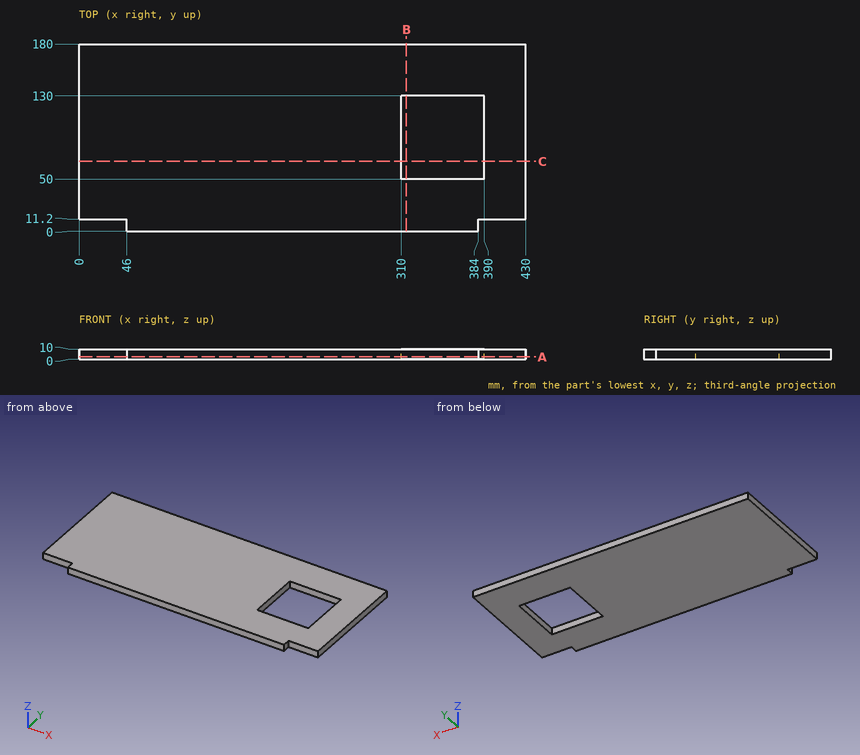
Drawing for the job (mm, zero at the part's lowest x, y, z). Give positions to 0.01 mm unless a question says otherwise; leave off trailing zeros. Order: outer loops, then holes, each group sorted by start corner. A loop starts at its lowest first (then second) coordinate and runs counter-clockwise, first axis right, second up. Notation, with made-up numbers: M -22.75,13 L 36.25,13 A17 ccw 36.25,41 Z; hole C 77,-32 d11. An arc over 180 degrees is marked long. Put each result on its own line as item: value. Start each with the question number.
(1) Drill centre lines: line 1 along X through (y, z) = (129, 6.5); line 2 along Y through (x, z) = (337.5, 5.75). Where is each one in solid material? Low to high.
(2) Saw through at B-B, the plane x = 315. Write the cut outline in (y, z).
(3) Saw through at C-C, the plane y = 67. Write the cut outline in (x, z), then the cut area to 3 significant figures.
(4) Saw through at A-A, the plane z = 2.5. Write the cut outline in (x, y), then the cut area to 3 significant figures.
(5) Flat gauge pin, fed straight in: pin 1 Ø3 at (y, z) = (88, 4) entering from -X. Where does the tip first touch, or does it go through?
Check result:
1. line 1: x = 0 to 310, 390 to 430
1. line 2: y = 0 to 50, 130 to 180
2. outline: M 0,0 L 50,0 L 50,10 L 0,10 Z; M 130,0 L 180,0 L 180,10 L 130,10 Z
3. outline: M 0,0 L 310,0 L 310,10 L 0,10 Z; M 390,0 L 430,0 L 430,10 L 390,10 Z
3. area: 3,500 mm2
4. outline: M 0,11.2 L 46,11.2 L 46,0 L 384,0 L 384,11.2 L 430,11.2 L 430,180 L 0,180 Z; hole M 310,50 L 390,50 L 390,130 L 310,130 Z
4. area: 70,000 mm2
5. pin 1: stops at x = 0
